from build123d import *

# Parameters (mm, degrees)
BOX_W     = 10
BOX_H     = 10
BOX_DEPTH = 1


with BuildPart() as cube:
    # Box → Box (new body)
    with BuildSketch(Plane(origin=(-5, -5, 0), x_dir=(1, 0, 0), z_dir=(0, 0, 1))):
        with Locations((5, 5)):
            Rectangle(BOX_W, BOX_H)
    extrude(amount=BOX_DEPTH)


with BuildPart() as cone:
    # Cone → Cone (revolve)
    with BuildSketch(Plane.XZ):
        Polygon((0, 0), (4, 0), (1, 10), (0, 10), align=None)
    revolve(axis=Axis((0, 0, 0), (0, 0, 1)))


with BuildPart() as fusion:
    # Cone001 → Cone001 (revolve)
    with BuildSketch(Plane.XZ):
        Polygon((0, 0), (4.3, 0), (1.3, 10), (0, 10), align=None)
    revolve(axis=Axis((0, 0, 0), (0, 0, 1)))

    # Cut: cut Cone
    add(cone.part, mode=Mode.SUBTRACT)


with BuildPart() as fusion_1:
    # Cut placement: moved
    add(fusion.part.moved(Location((0, 0, 1))))

    # Fusion: union Cube
    add(cube.part)


solid = fusion_1.part
Can you work these out from the model? Positions are in its coordinate system, mm. A direction names the side the tool comes from. Coordinates: 2 decimals unless noted, no trailing zeros. Order: outer loops, then holes, each group sorted by start corner. A loop starts at its lowest first (then second) coordinate and runs counter-clockwise, first axis right, second up. Notation, with made-up numbers: M 22.5,-29 L 38.5,-29 A14 ccw 38.5,-11 Z; hole C -8.75,83.5 d11. An arc over 180 degrees is marked long. Answer as CSV lines item,"result".
(1) Please list where these lines run through material, in increasing order: L1, parallel to Z at x = -2.75, y = 2.75; L2, parallel to X at y = -1.5, z = 7.5; L3, parallel to Z at x = 0, y = 0.75.
Geometry check:
L1,"0 to 1, 1.37 to 2.37"
L2,"-1.81 to -1.4, 1.4 to 1.81"
L3,"0 to 1"
(2) If we mould it in two halves opening along X, with no side actions, what happens to faces 4 (the flat face through (0, 0, 0)), 5 (the conical face through (-0.53, -2.39, 7.18)), 6 (the flat face through (0, 0, 1))? For each: released by +X, released by -X, zero draft, split by the parting line, or undercut.
Geometry check:
face 4,"zero draft"
face 5,"split by the parting line"
face 6,"undercut"
(3) On a 3-axis mill with a long thin cutter (end or side, diameter ignored), from which of +Z, -Z, +X, -X, +Y, -Y can I reach the whole of each face in a straight line? I mean faces 1 (the flat face through (-4.5, 0.1, 1)), 2 (the conical face through (-1.7, -1.3, 7.2)), 3 (the flat face through (-0.1, -5, 0.5)). Say none if no direction works.
Geometry check:
face 1,"+Z"
face 2,"none"
face 3,"+Z, -Z, +X, -X, -Y"
(4) Suppose I cut it at A-A on y = 0. Please give me the cut outline in (x, z), plus the area to 3 significant figures.
Geometry check:
outline,"M -5,0 L 5,0 L 5,1 L 4.3,1 L 1.3,11 L 1,11 L 4,1 L -4,1 L -1,11 L -1.3,11 L -4.3,1 L -5,1 Z"
area,"16.0 mm^2"
(5) Suppose I cut it at B-B on z = 9. Please give me the cut outline in (x, y).
Geometry check:
outline,"C 0,0 d3.8; hole C 0,0 d3.2"
(6) Suppose I cut it at D-D on z = 4. Please give me the cut outline in (x, y), plus the area to 3 significant figures.
Geometry check:
outline,"C 0,0 d6.8; hole C 0,0 d6.2"
area,"6.13 mm^2"
(7) I'm going to push flat-ended pins straight in: pin 1 (4 mm diameter, centred on x = 2.5, z = 9.5, fed in from +Y); pin 2 (1.5 mm diameter, centred on y = 2.5, z = 3, fed in from +X); pin 3 (1 mm diameter, centred on x = -1, y = -2.5, fed in from -Z); pin 4 (2 mm diameter, centred on y = 0.5, z = 6, fed in from -X). Where does each tip first touch, or does it pass through?
Geometry check:
pin 1,"y = 1.91"
pin 2,"x = 3.33"
pin 3,"z = 0"
pin 4,"x = -3.08"
